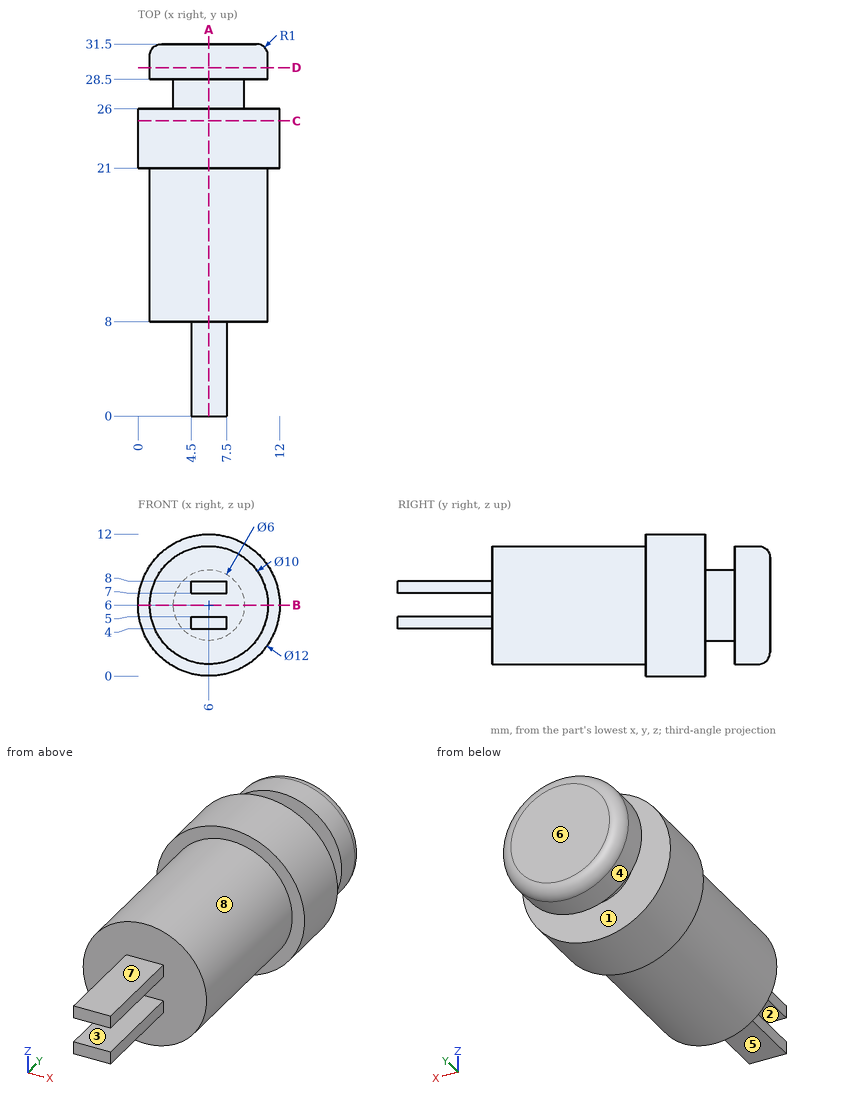
Verification items for this drawing (mm, ordinates from the low corner). A direction names the side the tool comes from. Give positions to 0.01 mm unless a question says otherwise; leave off trailing zeros. Loops run counter-clockwise (first coordinate to the right, second up) from the corner with the lowest first, then second, coordinate; pieces in that order, holes last. Notation, with made-up numbers: M 76,30 L 132,30 A25 cw 132,60 Z; hole C 16,89 d3. An arc over 180 degrees is marked long. Answer as CSV lines item,"result".
Item 1: Depth check by flat-ended pin: P1, Ø6, axis at x = 9, z = 6.5, coming from the -Y side; P2, Ø1.5, axis at x = 5.5, y = 3.5, coming from the +Z side; P3, Ø3, axis at x = 9, y = 24, coming from the +Z side; P4, Ø1.1, axis at y = 4.5, z = 7.5, coming from the -X side. Enter the tip coordinate at first touch or a pass-through.
Values:
P1,"stops at y = 0"
P2,"stops at z = 8"
P3,"stops at z = 11.81"
P4,"stops at x = 4.5"
Item 2: Cross-section at D-D on y = 29.5. Record the cut outline in (x, z), and give its area (3 significant figures).
Values:
outline,"C 6,6 d10"
area,"78.5 mm²"
Item 3: Access from +Z, -Z, +X, -X, +Y, -Y to the whole of each face (thin tool, end or side, straight path). Record for the marked faces 5, 6, 7 and 8.
Values:
face 5,"-Z, +X, -X, -Y"
face 6,"+Z, -Z, +X, -X, +Y"
face 7,"+Z, +X, -X, -Y"
face 8,"-Y"
Item 4: Material ranges on line 1 (Y direction, x = 7.75, z = 2.5); line 2 (Y direction, x = 4.75, z = 5.75); line 3 (Y direction, x = 5, z = 1), recorded low to high.
Values:
line 1,"y = 8 to 26, 28.5 to 31.5"
line 2,"y = 8 to 31.5"
line 3,"y = 21 to 26"
Item 5: Cross-section at C-C on y = 25. Record the cut outline in (x, z).
Values:
outline,"C 6,6 d12"
Item 6: Cross-section at B-B on z = 6. Record the cut outline in (x, y).
Values:
outline,"M 0,21 L 1,21 L 1,8 L 11,8 L 11,21 L 12,21 L 12,26 L 9,26 L 9,28.5 L 11,28.5 L 11,30.5 A1 ccw 10,31.5 L 2,31.5 A1 ccw 1,30.5 L 1,28.5 L 3,28.5 L 3,26 L 0,26 Z"
Item 7: Release check for a two-part mould opening along Z. For the marked faces 1, 2, 3 and 4 record: pulls with the +Z half, pulls with the -Z half, needs draft (parallel to the pull), parting line crosses it, or undercut.
Values:
face 1,"needs draft"
face 2,"undercut"
face 3,"undercut"
face 4,"parting line crosses it"
Item 8: Cross-section at A-A on x = 6. Record the cut outline in (y, z), and give its area (3 significant figures).
Values:
outline,"M 0,4 L 8,4 L 8,1 L 21,1 L 21,0 L 26,0 L 26,3 L 28.5,3 L 28.5,1 L 30.5,1 A1 ccw 31.5,2 L 31.5,10 A1 ccw 30.5,11 L 28.5,11 L 28.5,9 L 26,9 L 26,12 L 21,12 L 21,11 L 8,11 L 8,8 L 0,8 L 0,7 L 8,7 L 8,5 L 0,5 Z"
area,"251 mm²"
